Check sheet for the drawn part. Datum: minimum x, y, z corner. Units: mm. Round coordinates to 2 decimals unless told otherwise and drop trailing zeros. Write each loop counter-clockwise with the first axis right and the second up, starting at its lowest first coordinate (ties: lowest second). Pieces come first, ordered by that corner, then holes. Notation, with made-up numbers: M 1,21.25 L 10,21.25 A36 ccw 10,60.25 Z; hole C -0.75,1.25 d6. An arc over 180 degrees is marked long. One line per item, written item: value. Start each with the question number.
1. Depth check by flat-ended pin: P1, Ø1.5, axis at x = 81, z = 2, coming from the +Y side; P2, Ø1.5, axis at x = 86.5, z = 2, coming from the -Y side; P3, Ø1.5, axis at y = 3.5, z = 1, coming from the +X side. Enter the tip coordinate at first touch or a pass-through.
2. Section check A-A (y = 10). Record the boundary of the cut face in (x, z).
3. Scan lines: probe 1 along X at (y, z) = (42, 1.55); probe 2 along Y at (x, z) = (15, 1.6); probe 3 along Y at (x, z) = (51, 2.5). Record each from-to range of solid material in increasing order. Write a range as [from, to].
4. Section check B-B (z = 2.3). Record the boundary of the cut face in (x, y).
5. Section check D-D (x = 15). Record the boundary of the cut face in (y, z).
6. Section check C-C (y = 26.5). Record the boundary of the cut face in (x, z).
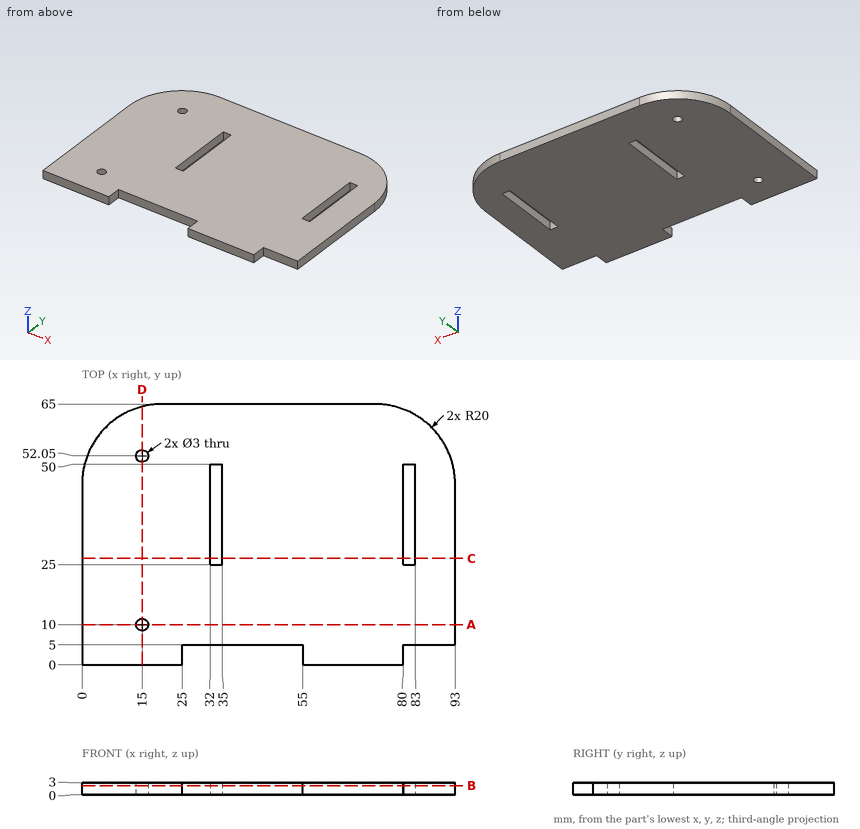
Result sheet:
1. P1: stops at y = 63.64
1. P2: stops at y = 5
1. P3: stops at x = 80
2. outline: M 0,0 L 13.5,0 L 13.5,3 L 0,3 Z; M 16.5,0 L 93,0 L 93,3 L 16.5,3 Z
3. probe 1: x = [0, 32], [35, 80], [83, 93]
3. probe 2: y = [0, 8.5], [11.5, 50.55], [53.55, 64.36]
3. probe 3: y = [5, 65]
4. outline: M 0,0 L 25,0 L 25,5 L 55,5 L 55,0 L 80,0 L 80,5 L 93,5 L 93,45 A20 ccw 73,65 L 20,65 A20 ccw 0,45 Z; hole C 15,10 d3; hole C 15,52.05 d3; hole M 32,25 L 35,25 L 35,50 L 32,50 Z; hole M 80,25 L 83,25 L 83,50 L 80,50 Z
5. outline: M 0,0 L 8.5,0 L 8.5,3 L 0,3 Z; M 11.5,0 L 50.55,0 L 50.55,3 L 11.5,3 Z; M 53.55,0 L 64.36,0 L 64.36,3 L 53.55,3 Z
6. outline: M 0,0 L 32,0 L 32,3 L 0,3 Z; M 35,0 L 80,0 L 80,3 L 35,3 Z; M 83,0 L 93,0 L 93,3 L 83,3 Z
